```python
from build123d import *

# Parameters (mm, degrees)
F5_DEPTH = 1.5
F6_SIZE  = 0.3
F7_R     = 0.2


with BuildPart() as f1:
    # F0 (on Front) → F1 (revolve)
    with BuildSketch(Plane.XZ):
        Polygon((3, 3), (0, 3), (0, -10), (1.5, -10), (1.5, 0), (3, 0), align=None)
    revolve(axis=Axis((0, 0, -3.5), (0, 0, 1)))

    # F2 (on Front) → F3 (revolve, cut)
    with BuildSketch(Plane.XZ):
        Polygon((1.515544, 3), (0, 3), (0, 0.778312), (1.25, 1.5), (1.25, 2.846688), align=None)
    revolve(axis=Axis((0, 0, 1.889156), (0, 0, -1)), mode=Mode.SUBTRACT)

    # F4 (on face) → F5 (cut)
    with BuildSketch(Plane.XY.offset(3)):
        Polygon((1.443376, 0), (0.721688, 1.25), (-0.721688, 1.25), (-1.443376, 0), (-0.721688, -1.25), (0.721688, -1.25), align=None)
    extrude(amount=-F5_DEPTH, mode=Mode.SUBTRACT)

    # F6
    f6_edges = [f1.edges().sort_by_distance(p)[0] for p in [
        (-3, 0, 3),
        (-1.5, 0, -10),
    ]]
    chamfer(f6_edges, length=F6_SIZE)

    # F7
    f7_edges = [f1.edges().sort_by_distance(p)[0] for p in [
        (-1.5, 0, 0),
    ]]
    fillet(f7_edges, radius=F7_R)


solid = f1.part
```
The model under review builds one solid part; all positions refer to its coordinate system, in mm. A direction names the side the tool comes from. Round coordinates to 2 decimals unless told otherwise and drop trailing zeros. Loops run counter-clockwise (first coordinate to the right, second up) from the corner with the lowest first, then second, coordinate; pieces in that order, holes last. Notation, with made-up numbers: (58.5, 66) -> (89.5, 66) arc R19 ccw to (89.5, 78) -> close; hole circle Ø3 at (49, 46). An arc over 180 degrees is marked (long way). Answer as a JSON object with one key per item and string values. Group by question number.
1) For pin 1 Ø0.7 at (x, y) = (-0.5, -1) entering from +Z; pin 2 Ø1.5 at (y, z) = (-1, -7.5) entering from +X; pin 3 Ø2 at (x, z) = (1.5, -3.5) entering from -Y, all flat-tipped, find the tip position at first contact; note any pin that passes through.
2) We need section A-A on z = -2.5. Write out the cut boundary in (x, y).
3) Mouldability with a two-part tool opening along X and no side actions: class faces 1 (the face through (-1.088, -0.616, 2.239)), 2 (the face through (-3, 0, 1)), 3 (the face through (0, -2, 0)) as released by +X, released by -X, zero draft, split by the parting line, or undercut.
4) For line 1 (Z direction, x = -2, y = -0.8); line 2 (X direction, y = 1.2, z = 1.75); line 3 (Y direction, x = -1.25, z = 2.25), list the stretches that pass through material, from the lowest coordinate up. Write a range as [from, to].
5) For faces 4 (the face through (0, 0, -10)), 5 (the face through (0, -1.25, 2)), 6 (the face through (-1.5, 0.07, -4.88)), list the 3-axis set-ups (+Z, -Z, +X, -X, +Y, -Y) from which the entire face can be reached by the end or side of a thin tool; tool diameter is ignored.
Result set:
{
 "1": {"pin 1": "z = 2.97", "pin 2": "x = 1.48", "pin 3": "y = -1.41"},
 "2": {"outline": "circle Ø3 at (0, 0)"},
 "3": {"face 1": "undercut", "face 2": "split by the parting line", "face 3": "zero draft"},
 "4": {"line 1": "[0, 3]", "line 2": "[-2.75, -0.75], [0.75, 2.75]", "line 3": "[-2.73, -0.33], [0.33, 2.73]"},
 "5": {"face 4": "-Z, +X, -X, +Y, -Y", "face 5": "+Z", "face 6": "-Z"}
}
